Autodesk Fusion 360 part; units mm, degrees
sketch "Sketch1" plane through (0, 0, 0) normal (0, 1, 0) x (1, 0, 0)
  circle A0 centre (0, 0) radius 1.4
  circle A1 centre (0, -30.9) radius 1.4
  line L0 (0, -30.9) -> (0, 0) construction
  line L1 (-26.5, -15.45) -> (26.5, -15.45) construction
  line L2 (26.5, -0.05) -> (-26.5, -0.05)
  line L3 (-26.5, -0.05) -> (-26.5, -30.85)
  line L4 (-26.5, -30.85) -> (26.5, -30.85)
  line L5 (26.5, -30.85) -> (26.5, -0.05)
  line L6 (26.5, -0.05) -> (-26.5, -30.85) construction
  line L7 (-26.5, -0.05) -> (26.5, -30.85) construction
  line L8 (0, -38.45) -> (0, 7.55) construction
  line L9 (-26.5, -30.85) -> (-12.5, -35.15)
  line L10 (-12.5, -35.15) -> (0, -35.15)
  line L11 (26.5, -30.85) -> (12.5, -35.15)
  arc A2 (-12.5, -35.15) -> (12.5, -35.15) centre (0, -13.1258) ccw
  line L12 (-26.5, -0.05) -> (-12.5, 4.25)
  arc A3 (12.5, 4.25) -> (-12.5, 4.25) centre (0, -17.7742) ccw
  line L13 (26.5, -0.05) -> (12.5, 4.25)
  point P0 (0, -15.45)
  point P1 (0, -15.45)
  point P2 (0, -15.45)
  point P3 (0, -15.45)
  dimension "d1" = 2.8
  dimension "d2" = 2.8
  dimension "d3" = 30.9
  dimension "d4" = 53
  dimension "d5" = 53
  dimension "d6" = 30.8
  dimension "d7" = 14
  dimension "d8" = 19.7
  dimension "d9" = 46
extrude "Extrude1" add sketch "Sketch1" along normal blind 4
hole "Hole1" at (0, 0, 30.9) at (0, 0, 0) direction (0, 1, 0) diameter 2.529 end through all
sketch "Sketch2" plane through (0, 4, 0) normal (0, 1, 0) x (-1, 0, 0)
  circle A0 centre (0, 30.9) radius 1.2645
  circle A1 centre (0, 0) radius 1.2645
  line L0 (-26.5, 30.85) -> (-26.5, 0.05)
  line L1 (-26.5, 0.05) -> (-12.5, -4.25)
  arc A2 (-12.5, -4.25) -> (12.5, -4.25) centre (0, 17.7742) ccw
  line L2 (12.5, -4.25) -> (26.5, 0.05)
  line L3 (26.5, 0.05) -> (26.5, 30.85)
  line L4 (26.5, 30.85) -> (12.5, 35.15)
  arc A3 (12.5, 35.15) -> (-12.5, 35.15) centre (0, 13.1258) ccw
  line L5 (-12.5, 35.15) -> (-26.5, 30.85)
  line L6 (-26.5, 30.85) -> (26.5, 30.85)
  line L7 (-26.5, 30.85) -> (26.5, 30.85)
  line L8 (26.5, 30.85) -> (26.5, 34.85)
  line L9 (26.5, 34.85) -> (-26.5, 34.85)
  line L10 (-26.5, 34.85) -> (-26.5, 30.85)
  circle A4 centre (0, 30.9) radius 2.5
  dimension "d20" = 4
  dimension "d21" = 5
extrude "Extrude2" add sketch "Sketch2" along normal blind 25 contours L4 L5 L6 L7 L9 A4
sketch "Sketch3" plane through (0, 0, 30.85) normal (0, 0, -1) x (1, 0, 0)
  line L0 (26.5, -4) -> (-26.5, -4)
  line L1 (-26.5, -4) -> (-26.5, -29)
  line L2 (-26.5, -29) -> (26.5, -29)
  line L3 (26.5, -29) -> (26.5, -4)
  line L4 (-26.5, -16.5) -> (26.5, -16.5)
  line L5 (-9, -16.5) -> (-9, -29)
  line L6 (9, -16.5) -> (9, -29)
  line L7 (26.5, -4) -> (2.4995, -4)
  line L8 (2.4995, -29) -> (26.5, -29)
  line L9 (26.5, -29) -> (26.5, -4)
  line L10 (2.4995, -4) -> (2.4995, -29)
  dimension "d18" = 17.5
  dimension "d19" = 17.5
hole "Hole2" at (-9, 16.5, 30.85) at (9, 16.5, 30.85) direction (0, 0, 1) diameter 4.5 depth 4 tip angle 118 countersink diameter 9.4 countersink angle 90
sketch "Sketch4" plane through (-26.5, 0, 0) normal (-1, 0, 0) x (0, -1, 0)
  line L0 (0, 0.05) -> (0, 30.85)
  line L1 (0, 30.85) -> (-4, 30.85)
  line L2 (-4, 30.85) -> (-4, 0.05)
  line L3 (-4, 0.05) -> (0, 0.05)
  line L4 (0, 30.85) -> (0, 35.15)
  line L5 (0, 35.15) -> (-4, 35.15)
  line L6 (-4, 35.15) -> (-4, 34.85)
  line L7 (-4, 34.85) -> (-29, 34.85)
  line L8 (-29, 34.85) -> (-29, 30.85)
  line L9 (-29, 30.85) -> (-4, 30.85)
  line L10 (-4, 30.85) -> (0, 30.85)
  line L11 (-29, 30.85) -> (-4, 0.05)
sketch "Sketch5" plane through (26.5, 0, 0) normal (1, 0, 0) x (0, 1, 0)
  line L0 (0, 30.85) -> (0, 0.05)
  line L1 (0, 0.05) -> (4, 0.05)
  line L2 (4, 0.05) -> (4, 30.85)
  line L3 (4, 30.85) -> (0, 30.85)
  line L4 (0, 35.15) -> (0, 30.85)
  line L5 (0, 30.85) -> (4, 30.85)
  line L6 (4, 30.85) -> (29, 30.85)
  line L7 (29, 30.85) -> (29, 34.85)
  line L8 (29, 34.85) -> (4, 34.85)
  line L9 (4, 34.85) -> (4, 35.15)
  line L10 (4, 35.15) -> (0, 35.15)
  line L11 (29, 30.85) -> (4, 0.05)
extrude "Extrude3" add sketch "Sketch5" against normal blind 4 contours L2 L6 L11
extrude "Extrude4" add sketch "Sketch4" against normal blind 4 contours L2 L9 L11
equation "d8 = ( 39.4 / 2 ) * 1 mm"
Verification items for the finished model (mm, model axes). A direction names the side the tool comes from. Round coordinates to 2 decimals unless told otherwise and drop trailing zeros. Write each loop counter-clockwise with the first axis right and the second up, starting at its lowest first coordinate (ties: lowest second). Pieces come first, ordered by that corner, then holes.
(1) Section check D-D (z = 28). Enter the section's corners in (x, y).
Returned:
outline: (-26.5, 0) - (26.5, 0) - (26.5, 26.69) - (22.5, 26.69) - (22.5, 4) - (-22.5, 4) - (-22.5, 26.69) - (-26.5, 26.69) - close
(2) Depth check by flat-ended pin: pin 1 Ø20.5 at (x, z) = (6.5, 18.5) entering from +Y; pin 2 Ø10 at (x, y) = (-8, 22) entering from -Z; pin 3 Ø2 at (x, y) = (-0.5, 5.5) entering from +Z. Enter the tip coordinate at first touch or a pass-through.
Returned:
pin 1: stops at y = 4
pin 2: stops at z = 30.85
pin 3: stops at z = 34.85
(3) Mould release check, pull along X, two halves, no side actions. Record for faces 1 (the flat face through (-22.5, 11, 23)), 2 (the flat face through (0, 4, 36)), 3 (the cylindrical face through (0.48, 2.03, 29.73)), 4 (the flat face through (19.6, 1.97, -2.07)): pulls with the +X half, pulls with the -X half, needs draft (parallel to the pull), parting line crosses it, or undercut.
Returned:
face 1: undercut
face 2: needs draft
face 3: undercut
face 4: pulls with the +X half
(4) Section check A-A (y = 16.5). Enter the section's corners in (x, z), plus the area to 3 significant figures.
Returned:
outline: (-26.5, 15.45) - (-22.5, 15.45) - (-22.5, 30.85) - (-13.7, 30.85) - (-11.25, 33.3) - (-11.25, 34.85) - (-13.48, 34.85) - (-26.5, 30.85) - close; (-6.75, 33.3) - (-4.3, 30.85) - (-2.5, 30.85) arc R2.5 cw (long way) to (2.5, 30.85) - (4.3, 30.85) - (6.75, 33.3) - (6.75, 34.85) - (-6.75, 34.85) - close; (11.25, 33.3) - (13.7, 30.85) - (22.5, 30.85) - (22.5, 15.45) - (26.5, 15.45) - (26.5, 30.85) - (13.48, 34.85) - (11.25, 34.85) - close
area: 225 mm2
(5) Material ranges on line 1 (Z direction, x = 0, y = 2.95); line 2 (Y direction, x = 9, z = 34); line 3 (X direction, y = 11.75, z = 15), recorded low to high.
Returned:
line 1: z = -7.55 to -1.26, 1.26 to 29.64, 32.16 to 38.45
line 2: y = 0 to 14.25, 18.75 to 29
line 3: x = -26.5 to -22.5, 22.5 to 26.5
(6) Section check B-B (x = 9). Enter the section's corners in (y, z), plus the area to 3 significant figures.
Returned:
outline: (0, -5.9) - (4, -5.9) - (4, 30.85) - (11.8, 30.85) - (14.25, 33.3) - (14.25, 34.85) - (4, 34.85) - (4, 36.8) - (0, 36.8) - close; (18.75, 33.3) - (21.2, 30.85) - (29, 30.85) - (29, 34.85) - (18.75, 34.85) - close
area: 247 mm2
(7) Access from +Z, -Z, +X, -X, +Y, -Y to the whole of each face (thin tool, end or side, straight path). Record for faces 5 (the cylindrical face through (0.18, 1.97, 38.45)), 6 (the flat face through (-15, 16, 30.85)), 7 (the flat face through (0, 16, 34.85)).
Returned:
face 5: +Z, +Y, -Y
face 6: -Z, +Y
face 7: +Z, +X, -X, +Y
(8) Section check C-C (y = 9). Enter the section's corners in (x, z), plus the area to 3 significant figures.
Returned:
outline: (-26.5, 6.21) - (-22.5, 6.21) - (-22.5, 30.85) - (-2.5, 30.85) arc R2.5 cw (long way) to (2.5, 30.85) - (22.5, 30.85) - (22.5, 6.21) - (26.5, 6.21) - (26.5, 30.85) - (13.48, 34.85) - (-13.48, 34.85) - (-26.5, 30.85) - close
area: 347 mm2
